Autodesk Inventor part; units mm, degrees
ref_plane "YZ Plane" through (0, 0, 0) normal (1, 0, 0) x (0, 1, 0)
ref_plane "XZ Plane" through (0, 0, 0) normal (0, 1, 0) x (-1, 0, 0)
ref_plane "XY Plane" through (0, 0, 0) normal (0, 0, 1) x (1, 0, 0)
sketch "Sketch1" plane through (0, 0, 0) normal (0, 1, 0) x (-1, 0, 0)
  line L0 (-152.4, 279.4) -> (152.4, 279.4)
  line L1 (152.4, 279.4) -> (152.4, -279.4)
  line L2 (152.4, -279.4) -> (-152.4, -279.4)
  line L3 (-152.4, -279.4) -> (-152.4, 279.4)
  line L4 (-152.4, 279.4) -> (152.4, -279.4) construction
  line L5 (152.4, 279.4) -> (-152.4, -279.4) construction
  line L6 (-146.05, 273.05) -> (146.05, 273.05)
  line L7 (146.05, 273.05) -> (146.05, -273.05)
  line L8 (146.05, -273.05) -> (-146.05, -273.05)
  line L9 (-146.05, -273.05) -> (-146.05, 273.05)
  line L10 (-146.05, 273.05) -> (146.05, -273.05) construction
  line L11 (146.05, 273.05) -> (-146.05, -273.05) construction
  point P0 (0, 0)
  dimension "d0" = 558.8
  dimension "d1" = 304.8
  dimension "d2" = 546.1
  dimension "d3" = 292.1
extrude "Extrusion1" add sketch "Sketch1" along normal blind 6.35 contours L6 L7 L8 L9
extrude "Extrusion2" add sketch "Sketch1" along normal blind 101.6
sketch "Sketch2" plane through (0, 0, 0) normal (0, -1, 0) x (1, 0, 0)
  line L0 (-50, 10) -> (50, 10)
  line L1 (50, 10) -> (50, -10)
  line L2 (50, -10) -> (-50, -10)
  line L3 (-50, -10) -> (-50, 10)
  line L4 (-50, 10) -> (50, -10) construction
  line L5 (50, 10) -> (-50, -10) construction
  point P0 (0, 0)
  dimension "d8" = 20
  dimension "d9" = 100
extrude "Extrusion3" add sketch "Sketch2" along normal blind 50
sketch "Sketch4" plane through (50, 0, -10) normal (0, 0, -1) x (-1, 0, 0)
  line L0 (202.4, 0) -> (-102.4, 0)
  line L1 (90, 0) -> (90, -40)
  line L2 (90, -40) -> (10, -40)
  line L3 (10, -40) -> (10, 0)
  line L4 (100, -50) -> (0, -50)
  line L5 (0, 0) -> (0, -50)
  line L6 (100, 0) -> (100, -50)
  point P0 (50, 0)
  point P1 (50, -40)
  point P2 (0, -25)
  dimension "d17" = 10
  dimension "d18" = 10
  dimension "d19" = 10
extrude "Extrusion5" cut sketch "Sketch4" against normal blind 50 contours L1 L2 L3 L0
properties part number "Blackout Box"
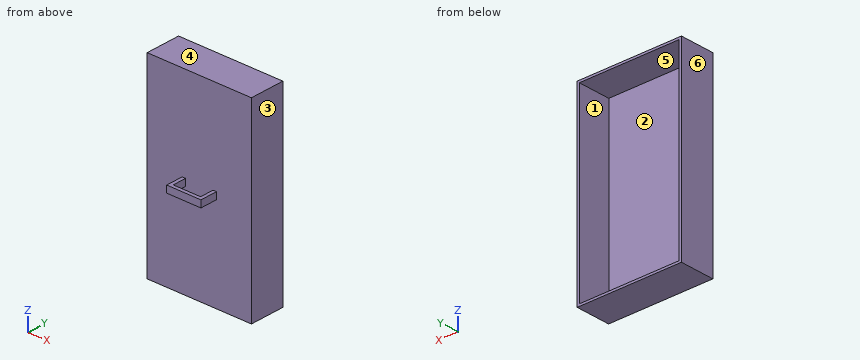
Build history of the part. All positions in model axes, mm. Face numbers are marked on the shaded views. A direction names the side the tool comes from. Give positions to 0.01 mm unless a question says otherwise; leave off trailing zeros. Order: outer loops, then holes, each group sorted by start corner. A loop starts at its lowest first (then second) coordinate and runs counter-clockwise, first axis right, second up. Notation, with made-up numbers: M 56.25,-23.5 L 74.25,-23.5 A11 cw 74.25,-19.5 Z; hole C -24,21.25 d2. An arc over 180 degrees is marked long. Put each result on its own line as item: value.
Item 1: Slice it at B-B, the plane z = 237. Write the cut outline in (x, y).
From the geometry:
outline: M -152.4,0 L 152.4,0 L 152.4,101.6 L 146.05,101.6 L 146.05,6.35 L -146.05,6.35 L -146.05,101.6 L -152.4,101.6 Z
Item 2: Probe line 1 (X direction, y = 56, z = -135); line 2 (Z direction, x = 70.5, y = 12); line 3 (Y direction, x = 122.5, z = 177). List the from-to ranges inside material, lowest first. Write a range as [from, to].
From the geometry:
line 1: x = [-152.4, -146.05], [146.05, 152.4]
line 2: z = [-279.4, -273.05], [273.05, 279.4]
line 3: y = [0, 6.35]
Item 3: Slice it at A-A, the plane x = 12.5. Write the cut outline in (y, z).
From the geometry:
outline: M -50,-10 L -40,-10 L -40,10 L -50,10 Z; M 0,-279.4 L 101.6,-279.4 L 101.6,-273.05 L 6.35,-273.05 L 6.35,273.05 L 101.6,273.05 L 101.6,279.4 L 0,279.4 Z
Item 4: Slice it at D-D, the plane z = 0. Write the cut outline in (x, y), plus the area to 3 significant figures.
From the geometry:
outline: M -152.4,0 L -50,0 L -50,-50 L 50,-50 L 50,0 L 152.4,0 L 152.4,101.6 L 146.05,101.6 L 146.05,6.35 L -146.05,6.35 L -146.05,101.6 L -152.4,101.6 Z; hole M -40,-40 L 40,-40 L 40,0 L -40,0 Z
area: 4,950 mm2
Item 5: Flat gauge pins, fed straight in: pin 1 Ø10 at (y, z) = (-25, 3) entering from +X; pin 2 Ø8 at (x, y) = (-97.5, -1.5) entering from +Z; pin 3 Ø6 at (x, z) = (-94, 59) entering from +Y; pin 4 Ø6 at (y, z) = (-28.5, -1) entering from -X. Where does each tip first touch, or does it go through?
From the geometry:
pin 1: stops at x = 50
pin 2: stops at z = 279.4
pin 3: stops at y = 6.35
pin 4: stops at x = -50
Item 6: 3-axis set-ups, long thin cutter, end or side, ignore diameter. For the marked faces 5 and 6: which of +Z, -Z, +X, -X, +Y, -Y reach the whole face in a straight line?
From the geometry:
face 5: +Y
face 6: +Z, -Z, -X, +Y, -Y
Item 7: Two-plate mould, pull along Z, no slides. Class the marked faces 1, 2, 3 and 4: +Z half, -Z half, draft (parallel to the pull), parting line (faces both ways), or undercut.
From the geometry:
face 1: undercut
face 2: undercut
face 3: draft
face 4: +Z half
Item 8: Slice it at C-C, the plane y = 39. Write the cut outline in (x, z).
From the geometry:
outline: M -152.4,-279.4 L 152.4,-279.4 L 152.4,279.4 L -152.4,279.4 Z; hole M -146.05,-273.05 L 146.05,-273.05 L 146.05,273.05 L -146.05,273.05 Z
